For this review, take the finished solid that the model builds, in its own axes (mm). A direction names the side the tool comes from. Round coordinates to 2 decimals unless told otherwise and drop trailing zeros. Order: outer loops, then holes, each group sorted by start corner. A loop starts at its lowest first (then second) coordinate and runs counter-clockwise, first axis right, second up. Notation, with made-up numbers: (87, 26) - (92, 26) arc R19 cw to (92, 38) - close; hole circle Ø6 at (-12.5, 26). An arc over 180 degrees is marked (long way). Write each question's results on one line, items separated by ' | '. Start each with the question number.
(1) Draft analysis for pull direction Y (two halves, no side actions). For faces 5 (the flat face through (0, -40, 5)), 6 (the flat face through (-40, 0, 5)), 7 (the flat face through (25, 10, 5)), 8 (the cylindrical face through (33.847, -0.766, 4.93)), state which applies: pulls with the +Y half, pulls with the -Y half, needs draft (parallel to the pull), parting line crosses it, or undercut.
(2) Take a section at A-A, the plane z = 3.5. Give the boundary of the cut face in (x, y).
(3) Take a section at D-D, the plane x = -1. Give the boundary of the cut face in (y, z), plus the area to 3 significant figures.
(4) Take a section at B-B, the plane x = -32. Give the boundary of the cut face in (y, z).
(5) Insertion check: pin 1 Ø12 at (x, y) = (19.5, -13.5) entering from +Z; pin 2 Ø5 at (x, z) = (-18, 6.5) entering from +Y; pin 3 Ø5 at (x, z) = (22, 7) entering from -Y; pin 4 Ø5 at (y, z) = (30.5, 3) entering from -X. Each pin has a flat end and moves straight along its axis. Give the tip position at first contact, or say it passes through.
(6) For L1, parallel to Y at x = 32, z = 6.5; L2, parallel to Y at x = 22, z = 5.5, list the stretches that pass through material, from the lowest coordinate up. Write a range as from..to.
(7) Take a section at C-C, the plane y = 0. Give the boundary of the cut face in (x, z).
(8) For faces 1 (the flat face through (10, -25, 5)), 2 (the flat face through (-10, -25, 5)), 3 (the flat face through (-25, 10, 5)), 4 (the flat face through (10, 25, 5)), list the 3-axis set-ups (+Z, -Z, +X, -X, +Y, -Y) from which the entire face can be reached by the end or side of a thin tool; tool diameter is ignored.
```python
from build123d import *

# Parameters (mm, degrees)
SKETCH_R  = 2
PAD_DEPTH = 10


with BuildPart() as part:
    # Sketch → Pad (new body)
    with BuildSketch(Plane.XY):
        Polygon((-10, 40), (10, 40), (10, 10), (40, 10), (40, -10), (10, -10), (10, -40), (-10, -40), (-10, -10), (-40, -10), (-40, 10), (-10, 10), align=None)
        with Locations((0, 32)):
            Circle(SKETCH_R, mode=Mode.SUBTRACT)
        with Locations((32, 0)):
            Circle(SKETCH_R, mode=Mode.SUBTRACT)
        with Locations((0, -32)):
            Circle(SKETCH_R, mode=Mode.SUBTRACT)
        with Locations((-32, 0)):
            Circle(SKETCH_R, mode=Mode.SUBTRACT)
    extrude(amount=PAD_DEPTH)


solid = part.part
```
Results below:
1) face 5: pulls with the -Y half | face 6: needs draft | face 7: pulls with the +Y half | face 8: undercut
2) outline: (-40, -10) - (-10, -10) - (-10, -40) - (10, -40) - (10, -10) - (40, -10) - (40, 10) - (10, 10) - (10, 40) - (-10, 40) - (-10, 10) - (-40, 10) - close; hole circle Ø4 at (-32, 0); hole circle Ø4 at (0, -32); hole circle Ø4 at (0, 32); hole circle Ø4 at (32, 0)
3) outline: (-40, 0) - (-33.73, 0) - (-33.73, 10) - (-40, 10) - close; (-30.27, 0) - (30.27, 0) - (30.27, 10) - (-30.27, 10) - close; (33.73, 0) - (40, 0) - (40, 10) - (33.73, 10) - close | area: 731 mm^2
4) outline: (-10, 0) - (-2, 0) - (-2, 10) - (-10, 10) - close; (2, 0) - (10, 0) - (10, 10) - (2, 10) - close
5) pin 1: stops at z = 10 | pin 2: stops at y = 10 | pin 3: stops at y = -10 | pin 4: stops at x = -10
6) L1: y = -10..-2, 2..10 | L2: y = -10..10
7) outline: (-40, 0) - (-34, 0) - (-34, 10) - (-40, 10) - close; (-30, 0) - (30, 0) - (30, 10) - (-30, 10) - close; (34, 0) - (40, 0) - (40, 10) - (34, 10) - close
8) face 1: +Z, -Z, +X, -Y | face 2: +Z, -Z, -X, -Y | face 3: +Z, -Z, -X, +Y | face 4: +Z, -Z, +X, +Y
